The listing builds one solid part. Answer for the finished solid, in the listing's coordinates (mm). Coordinates: 2 decimals unless noted, no trailing zeros. Loops run counter-clockwise (first coordinate to the right, second up) from the corner with the lowest first, then second, coordinate; pieces in that order, holes last. Notation, with made-up numbers: (13, -23) - (39, -23) arc R17 ccw to (39, 6) - close; hole circle Ø1 at (-9.5, 55.25). An arc over 180 degrees is marked (long way). One line per question, with ' | ' between items.
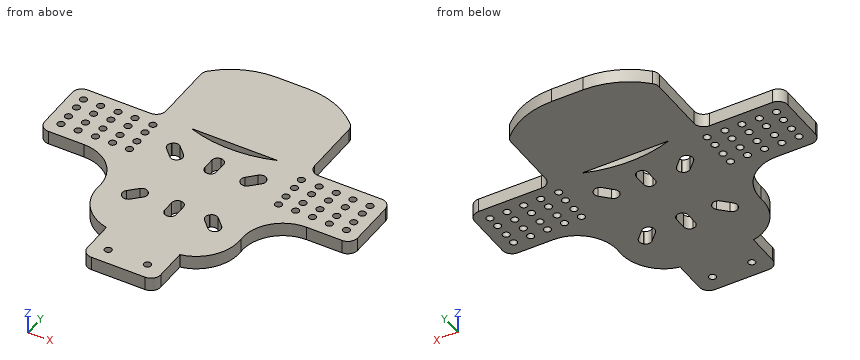
from build123d import *

# Parameters (mm, degrees)
F0_R        = 1.7924715581
F0_W        = 6
F0_H        = 12
F1_DEPTH    = 7
F2_R        = 5
F3_R        = 2.99999
F4_R        = 5
F5_R        = 5
F6_T1_DEPTH = 107.4648585932
F7_R        = 5
F8_R        = 5


# Not quite as in the source:
# - a fillet or chamfer that OpenCascade refuses, or shapes differently, is made with other operations: its cross-section is extruded or revolved along the edge and cut away or added
# - a fillet or chamfer is up to 0.001 mm smaller than in the source, because OpenCascade refuses the exact size


with BuildPart() as f1:
    # F0 (on Top) → F1 (new body)
    with BuildSketch(Plane.XY):
        with BuildLine():
            ThreePointArc((22.0503693582, 33.6896076798), (-0.0002403073, 29.9178496953), (-22.0508499728, 33.6896076798))
            Line((-22.0508499728, 33.6896076798), (-37.8788895905, 33.6896076798))
            Line((-37.8788895905, 33.6896076798), (-80, 33.6896076798))
            Line((-80, 33.6896076798), (-79.9124084099, -0.0643923202))
            Line((-79.9124084099, -0.0643923202), (-56.8817094834, -0.0643923202))
            ThreePointArc((-56.8817094834, -0.0643923202), (-41.9313295872, -6.4745981979), (-36.267593503, -21.72342412))
            ThreePointArc((-36.267593503, -21.72342412), (-31.9176063477, -36.6881030976), (-18.7309216708, -44.9932432158))
            Line((-18.7309216708, -44.9932432158), (-18.7309216708, -66.3649858077))
            Line((-18.7309216708, -66.3649858077), (0, -66.3649858077))
            Line((0, -66.3649858077), (18.7309216708, -66.3649858077))
            Line((18.7309216708, -66.3649858077), (18.7309216708, -44.9932432158))
            ThreePointArc((18.7309216708, -44.9932432158), (31.9176063477, -36.6881030976), (36.267593503, -21.72342412))
            ThreePointArc((36.267593503, -21.72342412), (41.9313295872, -6.4745981979), (56.8817094834, -0.0643923202))
            Line((56.8817094834, -0.0643923202), (79.9124084099, -0.0643923202))
            Line((79.9124084099, -0.0643923202), (80, 33.6896076798))
            Line((80, 33.6896076798), (37.8788895905, 33.6896076798))
            Line((37.8788895905, 33.6896076798), (22.0503693582, 33.6896076798))
        make_face()
        with Locations((-10.05, -58.1420399249)):
            Circle(F0_R, mode=Mode.SUBTRACT)
        with Locations((-72.8230625391, 7.1713337675)):
            Circle(F0_R, mode=Mode.SUBTRACT)
        with Locations((-64.1230625391, 7.1713337675)):
            Circle(F0_R, mode=Mode.SUBTRACT)
        with Locations((-55.4230625391, 7.4549200945)):
            Circle(F0_R, mode=Mode.SUBTRACT)
        with Locations((-46.7230625391, 7.4549200945)):
            Circle(F0_R, mode=Mode.SUBTRACT)
        Polygon((-22.0508499728, -24.7693415731), (-26.4349120161, -20.3852795298), (-17.9496306418, -11.8999981554), (-13.5655685985, -16.2840601989), align=None, mode=Mode.SUBTRACT)
        with Locations((-38.0230625391, 7.4549200945)):
            Circle(F0_R, mode=Mode.SUBTRACT)
        with Locations((10.05, -58.1420399249)):
            Circle(F0_R, mode=Mode.SUBTRACT)
        with Locations((0.059680174, -18.4716808143)):
            Rectangle(F0_W, F0_H, mode=Mode.SUBTRACT)
        Polygon((17.9491500272, -12.0967266704), (26.4344314015, -20.5820080448), (22.0503693582, -24.9660700881), (13.5650879839, -16.4807887139), align=None, mode=Mode.SUBTRACT)
        with Locations((38.0230625391, 7.4549200945)):
            Circle(F0_R, mode=Mode.SUBTRACT)
        with Locations((46.7230625391, 7.4549200945)):
            Circle(F0_R, mode=Mode.SUBTRACT)
        with Locations((55.4230625391, 7.4549200945)):
            Circle(F0_R, mode=Mode.SUBTRACT)
        with Locations((64.1230625391, 7.1713337675)):
            Circle(F0_R, mode=Mode.SUBTRACT)
        with Locations((72.8230625391, 7.1713337675)):
            Circle(F0_R, mode=Mode.SUBTRACT)
        with Locations((-72.8230625391, 13.522426948)):
            Circle(F0_R, mode=Mode.SUBTRACT)
        with Locations((-64.1230625391, 13.522426948)):
            Circle(F0_R, mode=Mode.SUBTRACT)
        with Locations((-72.9498788714, 20.6713337675)):
            Circle(F0_R, mode=Mode.SUBTRACT)
        with Locations((-73.1066465378, 27.022426948)):
            Circle(F0_R, mode=Mode.SUBTRACT)
        with Locations((-64.2498788714, 20.6713337675)):
            Circle(F0_R, mode=Mode.SUBTRACT)
        with Locations((-64.4066465378, 27.022426948)):
            Circle(F0_R, mode=Mode.SUBTRACT)
        with Locations((-55.4230625391, 13.8060132749)):
            Circle(F0_R, mode=Mode.SUBTRACT)
        with Locations((-46.7230625391, 13.8060132749)):
            Circle(F0_R, mode=Mode.SUBTRACT)
        with Locations((-55.5498788714, 20.9549200945)):
            Circle(F0_R, mode=Mode.SUBTRACT)
        with Locations((-55.7066465378, 27.3060132749)):
            Circle(F0_R, mode=Mode.SUBTRACT)
        with Locations((-46.8498788714, 20.9549200945)):
            Circle(F0_R, mode=Mode.SUBTRACT)
        with Locations((-47.0066465378, 27.3060132749)):
            Circle(F0_R, mode=Mode.SUBTRACT)
        with Locations((-38.0230625391, 13.8060132749)):
            Circle(F0_R, mode=Mode.SUBTRACT)
        Polygon((-13.5655685985, 14.0840613981), (-17.9496306418, 9.6999993546), (-26.4349120162, 18.185280729), (-22.0508499728, 22.5693427724), align=None, mode=Mode.SUBTRACT)
        with Locations((-38.1498788714, 20.9549200945)):
            Circle(F0_R, mode=Mode.SUBTRACT)
        with Locations((-37.8788895905, 27.3060132749)):
            Circle(F0_R, mode=Mode.SUBTRACT)
        with Locations((-0.0002403073, 16.1683102548)):
            Rectangle(F0_W, F0_H, mode=Mode.SUBTRACT)
        Polygon((22.0503693582, 22.7077228269), (26.4344314015, 18.1852813744), (17.9491500272, 9.7), (13.5650879839, 14.0840620435), align=None, mode=Mode.SUBTRACT)
        with Locations((38.0230625391, 13.8060132749)):
            Circle(F0_R, mode=Mode.SUBTRACT)
        with Locations((38.1498788714, 20.9549200945)):
            Circle(F0_R, mode=Mode.SUBTRACT)
        with Locations((37.8788895905, 27.3060132749)):
            Circle(F0_R, mode=Mode.SUBTRACT)
        with Locations((46.7230625391, 13.8060132749)):
            Circle(F0_R, mode=Mode.SUBTRACT)
        with Locations((55.4230625391, 13.8060132749)):
            Circle(F0_R, mode=Mode.SUBTRACT)
        with Locations((46.8498788714, 20.9549200945)):
            Circle(F0_R, mode=Mode.SUBTRACT)
        with Locations((47.0066465378, 27.3060132749)):
            Circle(F0_R, mode=Mode.SUBTRACT)
        with Locations((55.5498788714, 20.9549200945)):
            Circle(F0_R, mode=Mode.SUBTRACT)
        with Locations((55.7066465378, 27.3060132749)):
            Circle(F0_R, mode=Mode.SUBTRACT)
        with Locations((64.1230625391, 13.522426948)):
            Circle(F0_R, mode=Mode.SUBTRACT)
        with Locations((72.8230625391, 13.522426948)):
            Circle(F0_R, mode=Mode.SUBTRACT)
        with Locations((64.2498788714, 20.6713337675)):
            Circle(F0_R, mode=Mode.SUBTRACT)
        with Locations((64.4066465378, 27.022426948)):
            Circle(F0_R, mode=Mode.SUBTRACT)
        with Locations((72.9498788714, 20.6713337675)):
            Circle(F0_R, mode=Mode.SUBTRACT)
        with Locations((73.1066465378, 27.022426948)):
            Circle(F0_R, mode=Mode.SUBTRACT)
        Polygon((-37.8788895905, 33.6896076798), (-22.0508499728, 33.6896076798), (0, 33.6896076798), (0.149998191, 33.6896076798), (22.0503693582, 33.6896076798), (37.8788895905, 33.6896076798), (37.8788895905, 70.3556537628), (28.1570665538, 83.6896076798), (-28.1570665538, 83.6896076798), (-37.8788895905, 70.3556537628), align=None)
    extrude(amount=F1_DEPTH)

    # F2
    f2_edges = [f1.edges().sort_by_distance(p)[0] for p in [
        (-80, 33.689608, 3.5),
        (-79.912408, -0.064392, 3.5),
        (-18.730922, -66.364986, 3.5),
        (18.730922, -66.364986, 3.5),
        (79.912408, -0.064392, 3.5),
        (80, 33.689608, 3.5),
    ]]
    fillet(f2_edges, radius=F2_R)

    # F3 (radius 3 in the source; OpenCascade refuses exactly that, so slightly less here)
    f3_edges = [f1.edges().sort_by_distance(p)[0] for p in [
        (-22.05085, 22.569343, 3.5),
        (-13.565569, 14.084061, 3.5),
        (26.434431, 18.185281, 3.5),
        (22.050369, 22.707723, 3.5),
        (2.99976, 22.16831, 3.5),
        (-3.00024, 22.16831, 3.5),
        (-26.434912, 18.185281, 3.5),
        (-3.00024, 10.16831, 3.5),
        (-17.949631, 9.699999, 3.5),
        (17.94915, 9.7, 3.5),
        (13.565088, 14.084062, 3.5),
        (2.99976, 10.16831, 3.5),
        (13.565088, -16.480789, 3.5),
        (-2.94032, -24.471681, 3.5),
        (-2.94032, -12.471681, 3.5),
        (17.94915, -12.096727, 3.5),
        (3.05968, -12.471681, 3.5),
        (26.434431, -20.582008, 3.5),
        (22.050369, -24.96607, 3.5),
        (3.05968, -24.471681, 3.5),
        (-17.949631, -11.899998, 3.5),
        (-26.434912, -20.38528, 3.5),
        (-13.565569, -16.28406, 3.5),
        (-22.05085, -24.769342, 3.5),
    ]]
    fillet(f3_edges, radius=F3_R)

    # F4
    f4_edges = [f1.edges().sort_by_distance(p)[0] for p in [
        (-37.87889, 33.689608, 3.5),
    ]]
    fillet(f4_edges, radius=F4_R)

    # F5
    f5_edges = [f1.edges().sort_by_distance(p)[0] for p in [
        (37.87889, 33.689608, 3.5),
    ]]
    fillet(f5_edges, radius=F5_R)

    # F6: fillet of radius 40 on 2 edges, made by hand

    # F6_s2 → F6_t1 (cut)
    with BuildSketch(Plane.XY.offset(-50.2324292966)):
        with BuildLine():
            ThreePointArc((-8.0640948352, 83.6896076798), (-24.3944064777, 80.2042748926), (-37.8788895905, 70.3556537628))
            Line((-37.8788895905, 70.3556537628), (-28.1570665538, 83.6896076798))
            Line((-28.1570665538, 83.6896076798), (-8.0640948352, 83.6896076798))
        make_face()
        with BuildLine():
            ThreePointArc((37.8788895905, 70.3556537628), (24.3944064777, 80.2042748926), (8.0640948352, 83.6896076798))
            Line((8.0640948352, 83.6896076798), (28.1570665538, 83.6896076798))
            Line((28.1570665538, 83.6896076798), (37.8788895905, 70.3556537628))
        make_face()
    extrude(amount=F6_T1_DEPTH, mode=Mode.SUBTRACT)

    # F7
    f7_edges = [f1.edges().sort_by_distance(p)[0] for p in [
        (-37.87889, 70.355654, 3.5),
    ]]
    fillet(f7_edges, radius=F7_R)

    # F8
    f8_edges = [f1.edges().sort_by_distance(p)[0] for p in [
        (37.87889, 70.355654, 3.5),
    ]]
    fillet(f8_edges, radius=F8_R)


solid = f1.part
Item 1: Find the intervals of material crossed by line 1 (Y direction, x = 73, z = 3); line 2 (Y direction, x = 9.5, z = 5); line 3 (Y direction, x = -47, z = 3.5), in increasing order. Write a range as [from, to].
Taken from the geometry:
line 1: y = [-0.06, 5.39], [8.96, 11.74], [15.31, 18.88], [22.46, 25.23], [28.81, 33.69] | line 2: y = [-66.36, -59.85], [-56.44, 30.6], [33.69, 83.66] | line 3: y = [-2.58, 5.68], [9.23, 12.04], [15.58, 19.17], [22.74, 25.51], [29.1, 33.69]
Item 2: Find section B-B, the plane y = 48. Write down the section's boundary in (x, z), plus the area to 3 significant figures.
Taken from the geometry:
outline: (-37.88, 0) - (37.88, 0) - (37.88, 7) - (-37.88, 7) - close | area: 530 mm2
Item 3: Each of these flat-tipped pins is pushed along its axis until it touches: pin 1 Ø10 at (x, y) = (-44, -26) entering from -Z; pin 2 Ø2 at (x, z) = (57.5, 5) entering from +Y; pin 3 Ø4 at (x, y) = (-72.95, 20.67) entering from -Z; pin 4 Ø1.5 at (x, z) = (-52, 1.5) entering from -Y. Where does it stop, or does it pass through?
Taken from the geometry:
pin 1: passes through | pin 2: stops at y = 33.69 | pin 3: stops at z = 0 | pin 4: stops at y = -0.85
Item 4: Find section A-A, the plane x = 10.05. Write down the section's boundary in (y, z), plus the area to 3 significant figures.
Taken from the geometry:
outline: (-66.36, 0) - (-59.93, 0) - (-59.93, 7) - (-66.36, 7) - close; (-56.35, 0) - (30.68, 0) - (30.68, 7) - (-56.35, 7) - close; (33.69, 0) - (83.64, 0) - (83.64, 7) - (33.69, 7) - close | area: 1,000 mm2
Item 5: Find section D-D, the plane z = 1.5. State how many separate pieces and enclosed holes the cut face has, plus the area to 3 significant figures.
Taken from the geometry:
separate pieces: 1 | enclosed holes: 49 | area: 12,000 mm2
